```python
from build123d import *

# Parameters (mm, degrees)
BOSS_EXTRUDE1_DEPTH = 3.175
SKETCH2_W           = 1.27
SKETCH2_H           = 6.0452
CUT_EXTRUDE1_DEPTH  = 6.35
BOSS_EXTRUDE2_DEPTH = 5.715


with BuildPart() as part:
    # Sketch1 → Boss-Extrude1 (new, symmetric)
    with BuildSketch(Plane(origin=(0, 0, 0), x_dir=(1, 0, 0), z_dir=(0, 1, 0))):
        Polygon((20.32, 0), (16.51, 0), (16.51, 6.0452), (3.81, 6.0452), (3.81, 0), (0, 0), (0, -3.175), (20.32, -3.175), align=None)
        Polygon((3.175, 6.6802), (3.81, 6.0452), (5.715, 6.0452), (5.715, 9.2202), (4.699, 9.2202), (3.175, 7.6962), align=None)
        Polygon((14.605, 6.0452), (16.51, 6.0452), (17.145, 6.6802), (17.145, 7.6962), (15.621, 9.2202), (14.605, 9.2202), align=None)
        Polygon((3.81, 0), (16.51, 0), (20.32, 0), (20.32, -3.175), (0, -3.175), (0, 0), align=None)
    extrude(amount=BOSS_EXTRUDE1_DEPTH, both=True)

    # Sketch2 → Cut-Extrude1 (cut)
    with BuildSketch(Plane(origin=(0, 3.175, 0), x_dir=(1, 0, 0), z_dir=(0, 1, 0))):
        with Locations((6.35, 3.0226)):
            Rectangle(SKETCH2_W, SKETCH2_H)
        with Locations((13.97, 3.0226)):
            Rectangle(SKETCH2_W, SKETCH2_H)
    extrude(amount=-CUT_EXTRUDE1_DEPTH, mode=Mode.SUBTRACT)

    # Sketch1_3 → Boss-Extrude2 (add, symmetric)
    with BuildSketch(Plane(origin=(0, 0, 0), x_dir=(1, 0, 0), z_dir=(0, 1, 0))):
        Polygon((3.81, 0), (16.51, 0), (20.32, 0), (20.32, -3.175), (0, -3.175), (0, 0), align=None)
    extrude(amount=BOSS_EXTRUDE2_DEPTH, both=True)


solid = part.part
```
Build history of the part. All positions in model axes, mm. A direction names the side the tool comes from. Give positions to 0.01 mm unless a question says otherwise; leave off trailing zeros. Order: outer loops, then holes, each group sorted by start corner. A loop starts at its lowest first (then second) coordinate and runs counter-clockwise, first axis right, second up. Notation, with made-up numbers: M 78,-5.5 L 103,-5.5 A18 ccw 103,27.5 Z; hole C 10,66 d8. An arc over 180 degrees is marked long. Write item = value, one per line. Start each with the question number.
(1) Slice it at B-B on y = 0. Write the cut outline in (x, z) (3 decimals), plus the area to 3 significant figures.
(2) Two-plate mould, pull along X, no slides. Class faces 1 (the flat face through (3.175, 0, -7)), 2 (the flat face through (5.715, 0, -5)), 3 (the flat face through (15, 0, -9.22)), 4 (the flat face through (14.605, 0, -5)): released by +X, released by -X, zero draft, split by the parting line, or undercut.
(3) Pin check, flat tips, straight feed: pin 1 Ø2 at (x, z) = (15.5, -6) entering from -Y (3 decimals); pin 2 Ø1.5 at (x, z) = (14.5, -8) entering from +Y (3 decimals); pin 3 Ø1.8 at (y, z) = (-0.5, -3.5) entering from -X. Stop position of each tip, or through.
(4) Slice it at A-A on z = -2.75. Write the cut outline in (x, y) (3 decimals), plus the area to 3 significant figures.
(5) Probe L1, parallel to X at y = 3, z = -0.5 (3 decimals); L2, parallel to Z at x = 9.5, y = -5 (3 decimals); L3, parallel to Y at x = 12, z = -6 (3 decimals). List the from-to ranges inside material, lowest first. Write a range as [from, to].
(6) Slice it at C-C on x = 13. Write the cut outline in (y, z) (3 decimals), plus the area to 3 significant figures.
(7) Slice it at D-D on y = 4. Write the cut outline in (x, z) (3 decimals), plus the area to 3 significant figures.
(8) Which spindle directions (+Z, -Z, +X, -X, +Y, -Y) get a long thin tool onto all of the face, cutting with end or side? Do faces 5 (the flat face through (10, 0, -6.045)), 6 (the flat face through (5, 3.175, -5)), 7 (the flat face through (16.51, 0, -3)), 8 (the flat face through (16, -3.175, -5)). Say none if no direction does.
Responses:
q1.outline = M 0,0 L 3.81,0 L 3.81,-6.045 L 3.175,-6.68 L 3.175,-7.696 L 4.699,-9.22 L 5.715,-9.22 L 5.715,0 L 6.985,0 L 6.985,-6.045 L 13.335,-6.045 L 13.335,0 L 14.605,0 L 14.605,-9.22 L 15.621,-9.22 L 17.145,-7.696 L 17.145,-6.68 L 16.51,-6.045 L 16.51,0 L 20.32,0 L 20.32,3.175 L 0,3.175 Z
q1.area = 139 mm2
q2.face_1 = released by -X
q2.face_2 = undercut
q2.face_3 = zero draft
q2.face_4 = undercut
q3.pin_1 = -3.175
q3.pin_2 = 3.175
q3.pin_3 = 3.81
q4.outline = M 3.81,-3.175 L 5.715,-3.175 L 5.715,3.175 L 3.81,3.175 Z; M 6.985,-3.175 L 13.335,-3.175 L 13.335,3.175 L 6.985,3.175 Z; M 14.605,-3.175 L 16.51,-3.175 L 16.51,3.175 L 14.605,3.175 Z
q4.area = 64.5 mm2
q5.L1 = [3.81, 5.715], [6.985, 13.335], [14.605, 16.51]
q5.L2 = [0, 3.175]
q5.L3 = [-3.175, 3.175]
q6.outline = M -5.715,0 L -3.175,0 L -3.175,-6.045 L 3.175,-6.045 L 3.175,0 L 5.715,0 L 5.715,3.175 L -5.715,3.175 Z
q6.area = 74.7 mm2
q7.outline = M 0,0 L 20.32,0 L 20.32,3.175 L 0,3.175 Z
q7.area = 64.5 mm2
q8.face_5 = -Z, +Y, -Y
q8.face_6 = -Z, +X, -X, +Y
q8.face_7 = +X, +Y, -Y
q8.face_8 = -Z, +X, -X, -Y
